Autodesk Inventor part; units mm, degrees
ref_plane "Work Plane1" through (10.95, 0, 0) normal (0, 0, -1) x (1, 0, 0)
ref_plane "YZ Plane" through (0, 0, 0) normal (1, 0, 0) x (0, 1, 0)
ref_plane "XZ Plane" through (0, 0, 0) normal (0, 1, 0) x (-1, 0, 0)
sketch "Sketch1" plane through (0, 0, 0) normal (0, 0, 1) x (1, 0, 0)
  line L0 (-4.4577, 0) -> (-4.4577, 6.0778)
  line L1 (0, 8.763) -> (0, 4.7625)
  line L2 (2.3876, 4.7625) -> (15.875, 4.7625)
  line L3 (15.875, 4.7625) -> (15.875, 0)
  line L4 (15.875, 0) -> (-4.4577, 0)
  arc A0 (0, 8.763) -> (-2.9052, 9.4071) centre (-1.524, 8.763) ccw
  line L5 (0, -2.1146) -> (0, 12.6875)
  line L6 (-8.5242, 0) -> (19.9415, 0)
  line L7 (0, 4.7625) -> (0.0001, 4.7625)
  line L8 (0.0001, 4.7625) -> (0.0001, 4.7625)
  line L9 (0.0001, 4.7625) -> (0.7937, 4.7625)
  line L10 (0.7937, 4.7625) -> (2.3876, 4.7625)
  line L11 (-4.4577, 6.0778) -> (-2.9052, 9.4071)
  line L12 (0.0001, 4.7625) -> (2.3876, 4.7625) construction
  line L13 (2.3876, 4.7625) -> (2.3876, 0) construction
  dimension "d0" = 1.524
  dimension "d1" = 15.875
  dimension "d2" = 13.4874
  dimension "d3" = 20.574
  dimension "d4" = 9.525
  dimension "d5" = 4.4577
  dimension "d15" = 9.525
  dimension "d16" = 9.525
  dimension "d17" = 0.0001
  dimension "d18" = 1.5938
  dimension "d19" = 25
revolve "Body" add sketch "Sketch1" angle 360 about axis through (15.875, 0, 0) along (-1, 0, 0)
sketch "Sketch2" plane through (0, 0, 0) normal (1, 0, 0) x (0, 0, -1)
  line L0 (7.1438, 4.1244) -> (7.1437, -4.1244)
  line L1 (7.1437, -4.1244) -> (0, -8.2489)
  line L2 (0, -8.2489) -> (-7.1438, -4.1244)
  line L3 (-7.1438, -4.1244) -> (-7.1437, 4.1244)
  line L4 (-7.1437, 4.1244) -> (0, 8.2489)
  line L5 (0, 8.2489) -> (7.1438, 4.1244)
  point P0 (0, 0)
  point P1 (0, 0)
  dimension "d23" = 14.2875
extrude "Head" add sketch "Sketch2" against normal blind 9.906
sketch "Sketch3" plane through (0, 0, 0) normal (0, 0, 1) x (1, 0, 0)
  line L0 (-9.906, 7.1437) -> (-9.906, 8.2489)
  line L1 (-9.906, 8.2489) -> (-9.2679, 8.2489)
  line L2 (-9.2679, 8.2489) -> (-9.906, 7.1437)
  line L3 (-11.1981, 0) -> (-2.1531, 0)
  line L4 (-9.906, 8.2489) -> (-9.906, 4.1244)
  line L5 (-3.4453, 8.2489) -> (-9.906, 8.2489)
  point P0 (-9.906, 4.1244)
  dimension "d8" = 30
  dimension "d22" = 14.2875
revolve "Chamfer1" cut sketch "Sketch3" angle 360 about axis through (-10, 0, 0) along (1, 0, 0)
thread "Thread"
chamfer "Chamfer2" distance 0.9739 distance2 0.9739 1 edges at (15.875, -4.7625, 0) measured on face at (15.875, -1.4057, -0.0221)
ref_plane "Work Plane1" through (10.95, 0, 0) normal (0, 0, -1) x (1, 0, 0)
equation "\"d23\" = SW"
equation "\"d6\" = KOH"
equation "\"d10\" = GEL"
equation "\"d13\" = -0.5 * SPD + 0.5 * GD"
equation "\"d14\" = GUL"
equation "\"d0\" = PHH"
equation "\"d1\" = NLG"
equation "\"d2\" = GEL"
equation "\"d3\" = LADI"
equation "\"d4\" = GD"
equation "\"d5\" = 0.45 * KOH"
equation "\"d15\" = SD2"
equation "\"d16\" = BDM"
equation "\"d18\" = GAL"
equation "\"d19\" = KEWI"
equation "\"d8\" = ANG1"
equation "\"d22\" = SW0"
equation "\"NLG\" = 15.875"
equation "\"GD\" = NND"
equation "\"BDM\" = NND"
equation "\"KOH\" = 9.906"
equation "\"GEL\" = 13.4874"
equation "\"LADI\" = 20.574"
equation "\"SW\" = 14.2875"
equation "\"PHH\" = 1.524"
equation "\"SW0\" = SW"
equation "\"SPD\" = 7.5773"
equation "\"SD2\" = NND"
equation "\"SD\" = 0"
equation "\"ANG1\" = 30deg"
equation "\"KEWI\" = 25deg"
equation "\"GAL\" = 1.59385"
equation "\"GUL\" = 0.97385"
equation "\"THREADDIA\" = 9.525"
equation "\"SDH\" = SW"
equation "\"TOA\" = 30deg"
equation "\"NND\" = 9.525"
equation "\"E0\" = 1.155 * SW"
equation "\"GD1\" = 7.5773"
properties part number "92979A336" material "Steel, Mild"
Check sheet for the modelled part. Datum: model origin and axes. Units: mm. A direction names the side the tool comes from. Give positions to 0.01 mm unless a question says otherwise; leave off trailing zeros. Loops run counter-clockwise (first coordinate to the right, second up) from the corner with the lowest first, then second, coordinate; pieces in that order, holes last. Notation, with made-up numbers: (-34, -37.75) - (20, -37.75) arc R23 cw to (20, -23.75) - close; hole circle Ø7 at (68.5, -30.75). An arc over 180 degrees is marked (long way). One line per question, with ' | ' between items. Start each with the question number.
1. Cross-section at A-A, the plane x = -5.75. Enter the section's corners in (y, z).
2. Material ranges on line 1 along Y through (x, z) = (2, 0); line 2 along X through (y, z) = (-4.75, -2); line 3 along Z through (x, y) = (6.25, 3.5), recorded low to high. Write a range as [from, to].
3. Gauge pin test, flat ends, axial feed: pin 1 Ø1 at (y, z) = (4, -2.5) entering from +X; pin 2 Ø7 at (x, y) = (-6.5, 1) entering from +Z; pin 3 Ø12 at (x, z) = (10.5, -5.5) entering from +Y. Record the tip position at first contact, or that the pin passes through.
4. Set-up check for faces 1 (the flat face through (-6.63, -6.216, 3.522)), 2 (the flat face through (-6.63, 6.216, -3.522)), 3 (the flat face through (-6.63, 6.16, 3.62)), 4 (the flat face through (0, 4, 4)), 5 (the flat face through (-6.63, -6.16, -3.62)): record each of +Z, -Z, +X, -X, +Y, -Y from which the full face is reachable in a straight line by a thin tool's end or side.
5. Cross-section at B-B, the plane x = 9.5. Enter the section's corners in (y, z) (1 decimal).
Check result:
1) outline: (-8.25, 0) - (-4.12, -7.14) - (4.12, -7.14) - (8.25, 0) - (4.12, 7.14) - (-4.12, 7.14) - close
2) line 1: y = [-4.76, 4.76] | line 2: x = [-9.91, 0] | line 3: z = [-3.23, 3.23]
3) pin 1: stops at x = 15.45 | pin 2: stops at z = 9.16 | pin 3: stops at y = 4.76
4) face 1: +Z, -X, -Y | face 2: -Z, -X, +Y | face 3: +Z, -X, +Y | face 4: +X | face 5: -Z, -X, -Y
5) outline: circle Ø9.5 at (0, 0)
